The model under review builds one solid part; all positions refer to its coordinate system, in mm. A direction names the side the tool comes from. Coordinates: 2 decimals unless noted, no trailing zeros. Order: outer loops, then holes, each group sorted by start corner. A loop starts at its lowest first (then second) coordinate and runs counter-clockwise, first axis right, second up. Notation, with made-up numbers: M 51,81.25 L 110,81.25 A22 cw 110,117.25 Z; hole C 29,9.5 d10. An arc over 180 degrees is marked long. One line per item, written item: value.
```python
from build123d import *

# Parameters (mm, degrees)
BOSS_EXTRUDE1_DEPTH = 5.5
SKETCH1_3_R         = 12.749185426
SKETCH1_3_R_2       = 2.261632511
BOSS_EXTRUDE2_DEPTH = 8.5


with BuildPart() as part:
    # Sketch1 → Boss-Extrude1 (new body, symmetric)
    with BuildSketch(Plane.XY):
        with BuildLine():
            Line((10.968819498, -6.498209589), (46.22624128, -6.498209589))
            Line((46.22624128, -6.498209589), (46.22624128, 6.498209589))
            Line((46.22624128, 6.498209589), (10.968819498, 6.498209589))
            ThreePointArc((10.968819498, 6.498209589), (12.296040881, 3.36884367), (12.749185426, 0))
            ThreePointArc((12.749185426, 0), (12.296040881, -3.36884367), (10.968819498, -6.498209589))
        make_face()
    extrude(amount=BOSS_EXTRUDE1_DEPTH, both=True)

    # Sketch1_3 → Boss-Extrude2 (add, symmetric)
    with BuildSketch(Plane.XY):
        Circle(SKETCH1_3_R)
        Circle(SKETCH1_3_R_2, mode=Mode.SUBTRACT)
    extrude(amount=BOSS_EXTRUDE2_DEPTH, both=True)


solid = part.part
```
(1) For L1, parallel to Y at x = 0, z = 3.25; L2, parallel to Z at x = 15, y = -0.75; L3, parallel to Y at x = 24.5, z = 0.5, list the stretches that pass through material, from the lowest coordinate up.
Geometry results:
L1: y = -12.75 to -2.26, 2.26 to 12.75
L2: z = -5.5 to 5.5
L3: y = -6.5 to 6.5
(2) We need section B-B, the plane x = 0. State the section outline as (y, z) points.
Geometry results:
outline: M -12.75,-8.5 L -2.26,-8.5 L -2.26,8.5 L -12.75,8.5 Z; M 2.26,-8.5 L 12.75,-8.5 L 12.75,8.5 L 2.26,8.5 Z
(3) We need section C-C, the plane z = 0.5. State the section outline as (x, y) points, plus the area to 3 significant figures.
Geometry results:
outline: M 10.97,-6.5 L 46.23,-6.5 L 46.23,6.5 L 10.97,6.5 A12.75 ccw long Z; hole C 0,0 d4.52
area: 937 mm2
(4) We need section A-A, the plane y = 0. State the section outline as (x, z) points, plus the area to 3 significant figures.
Geometry results:
outline: M -12.75,-8.5 L -2.26,-8.5 L -2.26,8.5 L -12.75,8.5 Z; M 2.26,-8.5 L 12.75,-8.5 L 12.75,-5.5 L 46.23,-5.5 L 46.23,5.5 L 12.75,5.5 L 12.75,8.5 L 2.26,8.5 Z
area: 725 mm2
(5) We need section D-D, the plane y = -4. State the section outline as (x, z) points, plus the area to 3 significant figures.
Geometry results:
outline: M -12.11,-8.5 L 12.11,-8.5 L 12.11,-5.5 L 46.23,-5.5 L 46.23,5.5 L 12.11,5.5 L 12.11,8.5 L -12.11,8.5 Z
area: 787 mm2
(6) Insertion check: pin 1 Ø1.5 at (x, z) = (37.5, -5) entering from +Y; pin 2 Ø9 at (x, z) = (26.5, -0.5) entering from -Y; pin 3 Ø6.5 at (x, y) = (27, -3) entering from +Z; pin 4 Ø4 at (x, y) = (0, 0) entering from -Z. Each pin has a flat end and moves straight along its axis. Give the tip position at first contact, or say it passes through.
Geometry results:
pin 1: stops at y = 6.5
pin 2: stops at y = -6.5
pin 3: stops at z = 5.5
pin 4: passes through
(7) Mouldability with a two-part tool opening along Y and no side actions: class faces 3 (the flat face through (29, 6.498, 0)), 4 (the cylindrical face through (-0.49, -2.208, -0.119)), 5 (the flat face through (28, 0, 5.5)) as +Y half, -Y half, draft (parallel to the pull), parting line (faces both ways), or undercut.
Geometry results:
face 3: +Y half
face 4: undercut
face 5: draft
(8) Tool access review of faces 1 (the flat face through (28, -6.498, 0)), 2 (the flat face through (46.226, 0, 0)): name each direction out of +Z, -Z, +X, -X, +Y, -Y from which nothing blocks a thin tool from reaching the whole face with its end or side.
Geometry results:
face 1: +Z, -Z, +X, -Y
face 2: +Z, -Z, +X, +Y, -Y
